Study the drawing (mm; zero at the part's minimum x, y, z) and answer. A direction names the side the tool comes from. Coordinates: 2 decimals unless noted, no trailing zeros. Loops run counter-clockwise (first coordinate to the right, second up) from the corner with the lowest first, then second, coordinate; pieces in that order, holes last. Notation, with made-up numbers: (79.25, 9.25) -> (138.25, 9.25) arc R12 ccw to (138.25, 18.25) -> close; hole circle Ø10 at (2, 21). An arc over 180 degrees is marked (long way). Answer in a Markdown table with one row per item.
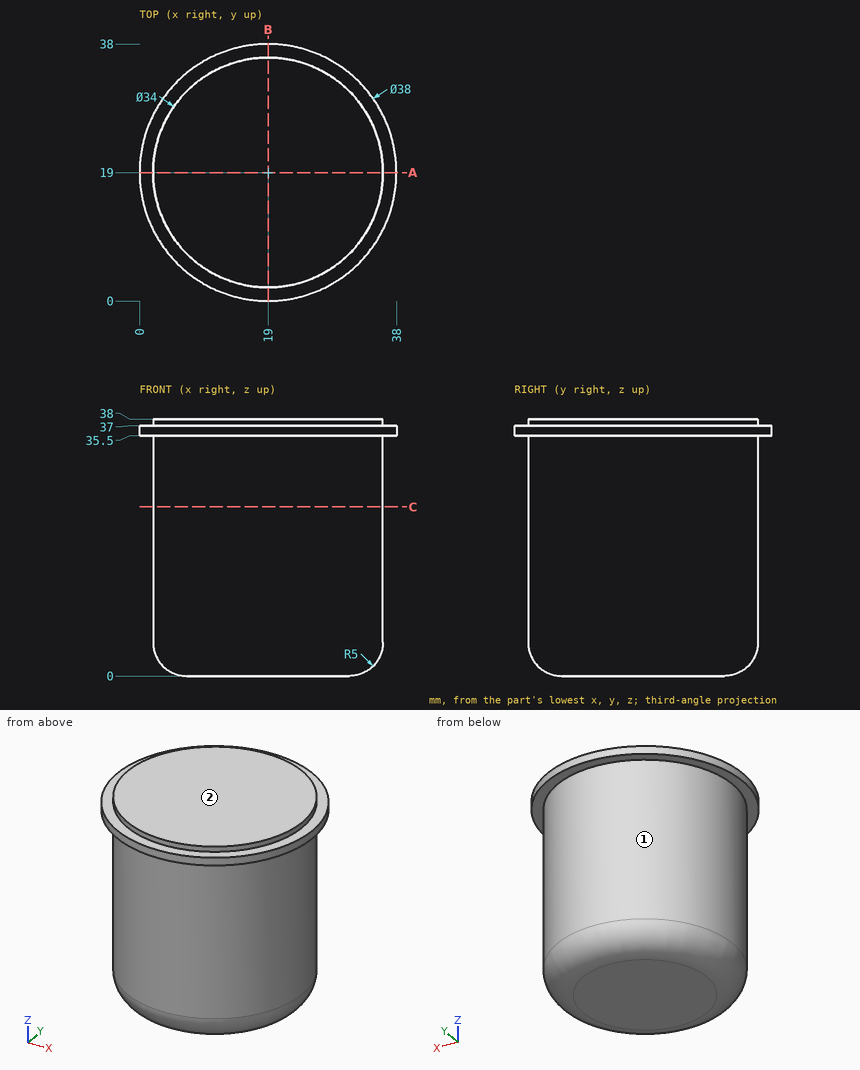
1. A cutting plane is placed at A-A on y = 19. Give the vertices of the cut face in (x, z), and give its area (3 significant figures).
A:
| item | result |
|---|---|
| outline | (0, 35.5) -> (2, 35.5) -> (2, 5) arc R5 ccw to (7, 0) -> (31, 0) arc R5 ccw to (36, 5) -> (36, 35.5) -> (38, 35.5) -> (38, 37) -> (36, 37) -> (36, 38) -> (2, 38) -> (2, 37) -> (0, 37) -> close |
| area | 1,290 mm2 |
2. A cutting plane is placed at C-C on z = 25. Give the vertices of the cut face in (x, y).
A:
| item | result |
|---|---|
| outline | circle Ø34 at (19, 19) |
3. A tool of negligible diameter and unlimited length cuts with its end or side. For the marked faces 1 and 2, from which of +Z, -Z, +X, -X, +Y, -Y can it reach the whole face along a straight path? Write none if from no direction.
A:
| item | result |
|---|---|
| face 1 | -Z |
| face 2 | +Z, +X, -X, +Y, -Y |
4. Given pin 1 Ø4 at (y, z) = (33, 15.5) entering from +X; pin 2 Ø5 at (x, z) = (24, 17.5) entering from +Y; pin 3 Ø1.5 at (y, z) = (29, 15.5) entering from -X, each flat-ended and moving along its own axis, determine where each tip first touches the part or whether it passes through.
A:
| item | result |
|---|---|
| pin 1 | stops at x = 31.04 |
| pin 2 | stops at y = 35.82 |
| pin 3 | stops at x = 4.74 |
5. Find the intervals of material crossed by probe 1 along X at (y, z) = (19.5, 13.5); probe 2 along X at (y, z) = (8, 10); probe 3 along Z at (x, y) = (30.5, 12.5), in increasing order.
A:
| item | result |
|---|---|
| probe 1 | x = 2.01 to 35.99 |
| probe 2 | x = 6.04 to 31.96 |
| probe 3 | z = 0.15 to 38 |
